The model under review builds one solid part; all positions refer to its coordinate system, in mm. A direction names the side the tool comes from. Give positions to 0.01 mm unless a question says otherwise; leave off trailing zeros. Order: outer loops, then holes, each group sorted by start corner. A loop starts at its lowest first (then second) coordinate and runs counter-clockwise, first axis right, second up.
```python
from build123d import *

# Parameters (mm, degrees)
EXTRUDE_THIN1_DEPTH = 12.5
BOSS_EXTRUDE1_DEPTH = 6
BOSS_EXTRUDE2_START = -12
BOSS_EXTRUDE2_DEPTH = 6
SKETCH4_R           = 9.5
CUT_EXTRUDE1_DEPTH  = 52.428062496


with BuildPart() as part:
    # Sketch1 → Extrude-Thin1 (new, symmetric)
    with BuildSketch(Plane.XY):
        Polygon((-35.921024484, 0), (-4.242640687, 0), (1.757359313, -6), (35.921024484, -6), (35.921024484, 0), (4.242640687, 0), (-1.757359313, 6), (-35.921024484, 6), align=None)
    extrude(amount=EXTRUDE_THIN1_DEPTH, both=True)

    # Sketch3 → Boss-Extrude1 (add)
    with BuildSketch(Plane(origin=(0, 6, 0), x_dir=(1, 0, 0), z_dir=(0, 1, 0))):
        with BuildLine():
            ThreePointArc((-35.921024484, 12.5), (-48.421024484, 0), (-35.921024484, -12.5))
            Line((-35.921024484, -12.5), (-35.921024484, 12.5))
        make_face()
    extrude(amount=-BOSS_EXTRUDE1_DEPTH)

    # Sketch3<3> → Boss-Extrude2 (add)
    with BuildSketch(Plane(origin=(0, 6, 0), x_dir=(1, 0, 0), z_dir=(0, 1, 0)).offset(BOSS_EXTRUDE2_START)):
        with BuildLine():
            Line((35.921024484, 12.5), (35.921024484, -12.5))
            ThreePointArc((35.921024484, -12.5), (48.421024484, 0), (35.921024484, 12.5))
        make_face()
    extrude(amount=BOSS_EXTRUDE2_DEPTH)

    # Sketch4 → Cut-Extrude1 (cut, through all)
    with BuildSketch(Plane(origin=(0, 6, 0), x_dir=(1, 0, 0), z_dir=(0, 1, 0))):
        with Locations(Location((-35.921024484, 0, 0), (0, 0, 180))):
            Circle(SKETCH4_R)
        with Locations(Location((35.921024484, 0, 0), (0, 0, 180))):
            Circle(SKETCH4_R)
    extrude(amount=-CUT_EXTRUDE1_DEPTH, mode=Mode.SUBTRACT)


solid = part.part
```
Item 1: Take a section at C-C (y = 1.75). Give the boundary of the cut face in (x, z), and give its area (3 significant figures).
Values found:
outline: (-35.92, -12.5) - (2.49, -12.5) - (2.49, 12.5) - (-35.92, 12.5) arc R12.5 ccw to start; hole circle Ø19 at (-35.92, 0)
area: 922 mm2
Item 2: Take a section at B-B (x = -35). Give the boundary of the cut face in (y, z).
Values found:
outline: (0, -12.5) - (6, -12.5) - (6, -9.46) - (0, -9.46) - close; (0, 9.46) - (6, 9.46) - (6, 12.5) - (0, 12.5) - close
Item 3: For line 1 (Y direction, x = -5, z = -1); line 2 (Y direction, x = 7, z = 2.5); line 3 (X direction, y = -3.5, z = 4), list the stretches that pass through material, from the lowest coordinate up.
Values found:
line 1: y = 0 to 6
line 2: y = -6 to 0
line 3: x = -0.74 to 27.3, 44.54 to 47.76
Item 4: Take a section at A-A (z = 0). Give the boundary of the cut face in (x, y), and give its area (3 significant figures).
Values found:
outline: (-48.42, 0) - (-45.42, 0) - (-45.42, 6) - (-48.42, 6) - close; (-26.42, 0) - (-4.24, 0) - (1.76, -6) - (26.42, -6) - (26.42, 0) - (4.24, 0) - (-1.76, 6) - (-26.42, 6) - close; (45.42, -6) - (48.42, -6) - (48.42, 0) - (45.42, 0) - close
area: 368 mm2
Item 5: Draft analysis for pull direction Z (two halves, no side actions). For faces 1 (the cylindrical face through (48.42, -3.04, 0.27)), 2 (the cylindrical face through (-26.43, 3.04, 0.42)), 3 (the flat face through (-1.28, -2.96, 0.18)), state which applies: released by +Z, released by -Z, zero draft, split by the parting line, or undercut.
Values found:
face 1: split by the parting line
face 2: undercut
face 3: zero draft
Item 6: For faces 4 (the flat face through (-22, 0, 0)), 5 (the flat face through (20, -6, 0)), 6 (the flat face through (21, 0, 0)), list the 3-axis set-ups (+Z, -Z, +X, -X, +Y, -Y) from which the entire face can be reached by the end or side of a thin tool; tool diameter is ignored.
Values found:
face 4: +Z, -Z, -X, -Y
face 5: +Z, -Z, +X, -X, -Y
face 6: +Z, -Z, +X, +Y
Item 7: Take a section at D-D (z = 5.75). Give the boundary of the cut face in (x, y).
Values found:
outline: (-47.02, 0) - (-43.48, 0) - (-43.48, 6) - (-47.02, 6) - close; (-28.36, 0) - (-4.24, 0) - (1.76, -6) - (28.36, -6) - (28.36, 0) - (4.24, 0) - (-1.76, 6) - (-28.36, 6) - close; (43.48, -6) - (47.02, -6) - (47.02, 0) - (43.48, 0) - close
Item 8: Clearance check with flat-ended pins moving along their axes: pin 1 Ø7.5 at (x, z) = (-25, 2) entering from -Y; pin 2 Ø1 at (y, z) = (-4, 6) entering from +X; pin 3 Ø4 at (x, y) = (-5, -4.5) entering from -Z. State where each tip first meets the part, or that it passes through.
Values found:
pin 1: stops at y = 0
pin 2: stops at x = 47.15
pin 3: passes through
